Can you work these out from the model? Positions are in its coordinate system, mm. A direction names the side the tool comes from. Coordinates: 2 decimals unless noted, no trailing zeros. Loops run counter-clockwise (first coordinate to the right, second up) from the corner with the lowest first, then second, coordinate; pieces in that order, holes last.
Autodesk Inventor part; units mm, degrees
ref_plane "YZ Plane" through (0, 0, 0) normal (1, 0, 0) x (0, 1, 0)
ref_plane "XZ Plane" through (0, 0, 0) normal (0, 1, 0) x (-1, 0, 0)
ref_plane "XY Plane" through (0, 0, 0) normal (0, 0, 1) x (1, 0, 0)
sketch "Sketch2" plane through (0, 0, 0) normal (0, 1, 0) x (-1, 0, 0)
  line L0 (-15, 12) -> (15, 12)
  line L1 (15, 12) -> (15, -12)
  line L2 (15, -12) -> (-15, -12)
  line L3 (-15, -12) -> (-15, 12)
  line L4 (-15, 12) -> (15, -12) construction
  line L5 (15, 12) -> (-15, -12) construction
  point P0 (0, 0)
  dimension "d5" = 30
  dimension "d6" = 24
extrude "Extrusion2" add sketch "Sketch2" along normal blind 4
sketch "Sketch3" plane through (0, 0, 0) normal (0, -1, 0) x (1, 0, 0)
  line L0 (-15, 12) -> (15, 12)
  line L1 (15, 12) -> (-15, 12)
  line L2 (-15, 12) -> (-15, 8)
  line L3 (-15, 8) -> (15, 8)
  line L4 (15, 8) -> (15, 12)
  line L5 (15, -12) -> (-15, -12)
  line L6 (-15, -12) -> (15, -12)
  line L7 (15, -12) -> (15, -8)
  line L8 (15, -8) -> (-15, -8)
  line L9 (-15, -8) -> (-15, -12)
  point P0 (0, 0)
  dimension "d9" = 4
  dimension "d10" = 4
extrude "Extrusion3" add sketch "Sketch3" along normal blind 54
sketch "Sketch4" plane through (-15, 4, 12) normal (0, 0, 1) x (1, 0, 0)
  line L0 (0, -58) -> (30, -58)
  line L1 (30, -4) -> (30, -58)
  line L2 (0, -58) -> (30, -58)
  line L3 (30, -58) -> (30, -54)
  line L4 (30, -54) -> (0, -54)
  line L5 (0, -54) -> (0, -58)
  point P0 (15, -4)
  dimension "d13" = 4
extrude "Extrusion4" add sketch "Sketch4" along normal blind 15
ref_plane "Work Plane1" through (-15, 0, 0) normal (0, 0, 1) x (1, 0, 0)
sketch "Sketch5" plane through (0, 4, 0) normal (0, 1, 0) x (1, 0, 0)
  line L0 (15, -8) -> (15, -27) construction
  line L1 (-15, 12) -> (15, 12) construction
  line L2 (15, -12.0945) -> (-15, 12) construction
  line L3 (-15, 12) -> (15, 12) construction
  line L4 (15, 12) -> (-15, -12.0945) construction
  circle A0 centre (0, 0) radius 6.731
  dimension "d16" = 13.462
extrude "Extrusion5" cut sketch "Sketch5" against normal blind 15.1625
sketch "Sketch6" plane through (-15, -50, 12) normal (0, 1, 0) x (1, 0, 0)
  line L0 (30, -15) -> (0, -15) construction
  line L1 (15, -15) -> (15, -8) construction
  point P0 (15, 12)
  dimension "d19" = 7
hole "Hole1" at (0, -50, 20) direction (0, -1, 0) diameter 4 end through all countersink diameter 8.5 countersink angle 82
sketch "Sketch7" plane through (-15, 4, -12) normal (-1, 0, 0) x (0, 0, 1)
  line L0 (24, -54) -> (39, -54)
  line L1 (24, -54) -> (24, 0)
  line L2 (39, -54) -> (24, 0)
  line L3 (24, 0) -> (24, -54)
  line L4 (24, -54) -> (39, -54)
  point P0 (12, -4)
extrude "Extrusion6" add sketch "Sketch7" against normal blind 5
mirror "Mirror1" about plane through (-15, 0, 0) normal (0, 0, 1) of "Hole1", "Extrusion6", "Extrusion4"
fillet "Fillet2" radius 3.175 4 edges at (2.5, 4, -12) (-12.5, 4, -12) (2.5, 4, 12) (-12.5, 4, 12)
sketch "Sketch8" plane through (0, -54, 0) normal (0, -1, 0) x (1, 0, 0)
  line L0 (15, 8) -> (15, 27)
  line L1 (-15, 8) -> (15, 8)
  line L2 (15, 27) -> (-15, 27)
  line L3 (-15, 27) -> (-15, 8)
  line L4 (-15, 8) -> (15, 8)
  line L5 (15, 8) -> (15, 27)
  line L6 (15, 8) -> (15, -8)
  line L7 (-10, -27) -> (-15, -27)
  line L8 (15, -8) -> (-15, -8)
  line L9 (-15, -8) -> (-15, -27)
  line L10 (-15, -27) -> (15, -27)
  line L11 (15, -27) -> (15, -8)
  circle A0 centre (0, 20) radius 2
  line L12 (-15, 8) -> (-15, 27)
  line L13 (-15, 8) -> (15, 8)
  line L14 (15, 8) -> (15, 27)
  line L15 (-15, 27) -> (15, 27)
  circle A1 centre (0, 20) radius 2
  circle A2 centre (0, -20) radius 2
  point P0 (0, 0)
extrude "Extrusion7" add sketch "Sketch8" along normal blind 3
properties part number "Main Power Switch Bracket"
(1) I want a section at A-A on x = 0. State how many separate pieces and enclosed holes the cut face has, then the cut area to 3 significant figures.
Check values:
separate pieces: 4
enclosed holes: 0
area: 636 mm2
(2) I want a section at C-C on y = -1. Write out the boundary of the cut face in (x, z).
Check values:
outline: (-15, -13.39) - (-10, -13.39) - (-10, -12) - (15, -12) - (15, -8) - (-15, -8) - close; (-15, 8) - (15, 8) - (15, 12) - (-10, 12) - (-10, 13.39) - (-15, 13.39) - close
(3) I want a section at D-D on z = 20. Write out the boundary of the cut face in (x, y).
Check values:
outline: (-15, -57) - (-2, -57) - (-2, -52.59) - (-4.25, -50) - (-10, -50) - (-10, -24.8) - (-15, -24.8) - close; (2, -57) - (15, -57) - (15, -50) - (4.25, -50) - (2, -52.59) - close
(4) I'm going to push flat-ended pins straight in: pin 1 (14.5 mm diameter, centred on y = -34, z = 17, fed in from +X); pin 2 (12.5 mm diameter, centred on x = 6.5, y = -21, fed in from +Z); pin 3 (1.5 mm diameter, centred on x = 11.5, z = -20.5, fed in from +Y); pin 4 (12.5 mm diameter, centred on x = -3.5, y = -35.5, fed in from -Z). Where does each tip first touch, or does it pass through?
Check values:
pin 1: stops at x = 15
pin 2: stops at z = 12
pin 3: stops at y = -50
pin 4: stops at z = -12
(5) I want a section at B-B on z = 0. Write out the boundary of the cut face in (x, y).
Check values:
outline: (-15, 0) - (-6.73, 0) - (-6.73, 4) - (-15, 4) - close; (6.73, 0) - (15, 0) - (15, 4) - (6.73, 4) - close
(6) Which directions (+Z, -Z, +X, -X, +Y, -Y) give clear straight access to the entire face, cutting with the end or side of a thin tool? Please do faces 1 (the flat face through (0, -28, -8)), 2 (the flat face through (2, -25, -12)), 3 (the cylindrical face through (2.68, 3.09, 11.05)).
Check values:
face 1: +X, -X, -Y
face 2: -Z, +X, +Y
face 3: +Z, +X, +Y
(7) If I drill on probe 1 along Z at (x, y) = (0, -54.65); probe 2 along Z at (x, y) = (0.5, -6); probe 3 along X at (y, z) = (-55.6, -20), over which ranges is the centre line in solid material (lowest first)?
Check values:
probe 1: z = -27 to -22, -18 to -8, 8 to 18, 22 to 27
probe 2: z = -12 to -8, 8 to 12
probe 3: x = -15 to -2, 2 to 15
